```python
from build123d import *

# Parameters (mm, degrees)
SKETCH3_W             = 152.4
SKETCH3_H             = 152.4
BOSS_EXTRUDE3_DEPTH   = 3.175
SKETCH13_R            = 7.5
CUT_EXTRUDE5_DEPTH    = 4.175
SKETCH15_R            = 1
CUT_EXTRUDE6_DEPTH    = 4.175
SKETCH17_W            = 12
SKETCH17_H            = 10.5
CUT_EXTRUDE7_DEPTH    = 4.175
FILLET1_R             = 3
SKETCH19_R            = 1.05
CUT_EXTRUDE8_DEPTH    = 4.175
SKETCH20_R            = 2.9718
BOLT_HOLES_DEPTH      = 1
BOLT_HOLES_DEPTH_BACK = 4.175
CUT_EXTRUDE12_DEPTH   = 3.175
FILLET2_R             = 6.35
MIRROR5_COPY_1_DEPTH  = 3.175
FILLET3_R             = 6.35
FILLET4_R             = 6.35


with BuildPart() as part:
    # Sketch3 → Boss-Extrude3 (new body)
    with BuildSketch(Plane.XY):
        Rectangle(SKETCH3_W, SKETCH3_H)
    extrude(amount=BOSS_EXTRUDE3_DEPTH)

    # Sketch13 → Cut-Extrude5 (cut, through all)
    with BuildSketch(Plane(origin=(0.106889783, -2.03090588, 3.175), x_dir=(1, 0, 0), z_dir=(0, 0, 1))):
        Circle(SKETCH13_R)
    extrude(amount=-CUT_EXTRUDE5_DEPTH, mode=Mode.SUBTRACT)

    # Sketch15 → Cut-Extrude6 (cut, through all)
    with BuildSketch(Plane(origin=(0.106889783, -2.03090588, 3.175), x_dir=(1, 0, 0), z_dir=(0, 0, 1))):
        with Locations((-28.5, -28.5)):
            Circle(SKETCH15_R)
        with Locations((-28.5, 28.5)):
            Circle(SKETCH15_R)
        with Locations((28.5, -28.5)):
            Circle(SKETCH15_R)
        with Locations((28.5, 28.5)):
            Circle(SKETCH15_R)
    extrude(amount=-CUT_EXTRUDE6_DEPTH, mode=Mode.SUBTRACT)

    # Sketch17 → Cut-Extrude7 (cut, through all)
    with BuildSketch(Plane(origin=(0.106889783, -2.03090588, 3.175), x_dir=(1, 0, 0), z_dir=(0, 0, 1))):
        with Locations((6, 0.25)):
            Rectangle(SKETCH17_W, SKETCH17_H)
    extrude(amount=-CUT_EXTRUDE7_DEPTH, mode=Mode.SUBTRACT)

    # Fillet1
    fillet1_edges = [part.edges().sort_by_distance(p)[0] for p in [
        (12.106889783, -7.03090588, 1.5875),
        (12.106889783, 3.46909412, 1.5875),
    ]]
    fillet(fillet1_edges, radius=FILLET1_R)

    # Sketch19 → Cut-Extrude8 (cut, through all)
    with BuildSketch(Plane(origin=(0.106889783, -2.03090588, 3.175), x_dir=(1, 0, 0), z_dir=(0, 0, 1))):
        with Locations((6.72, 6.72)):
            Circle(SKETCH19_R)
        with Locations((-6.72, 6.72)):
            Circle(SKETCH19_R)
        with Locations((-6.72, -6.72)):
            Circle(SKETCH19_R)
        with Locations((6.72, -6.72)):
            Circle(SKETCH19_R)
        with Locations((0, 10)):
            Circle(SKETCH19_R)
        with Locations((-10, 0)):
            Circle(SKETCH19_R)
        with Locations((0, -10)):
            Circle(SKETCH19_R)
    extrude(amount=-CUT_EXTRUDE8_DEPTH, mode=Mode.SUBTRACT)

    # Sketch20 → Bolt Holes (cut, two sides)
    with BuildSketch(Plane.XY.offset(3.175)) as bolt_holes_sk:
        with Locations((-69.83, 69.83)):
            Circle(SKETCH20_R)
        with Locations((69.83, 69.83)):
            Circle(SKETCH20_R)
        with Locations((69.83, -69.83)):
            Circle(SKETCH20_R)
        with Locations((-69.83, -69.83)):
            Circle(SKETCH20_R)
    extrude(amount=BOLT_HOLES_DEPTH, mode=Mode.SUBTRACT)
    extrude(bolt_holes_sk.sketch, amount=-BOLT_HOLES_DEPTH_BACK, mode=Mode.SUBTRACT)

    # Sketch25 → Cut-Extrude12 (cut)
    with BuildSketch(Plane.XY.offset(3.175)):
        with BuildLine():
            Line((-76.2, 50.8), (-76.2, -50.8))
            ThreePointArc((-76.2, -50.8), (-46.628854397, 0), (-76.2, 50.8))
        make_face()
    cut_extrude12 = extrude(amount=-CUT_EXTRUDE12_DEPTH, mode=Mode.SUBTRACT)

    # Fillet2
    fillet2_edges = [part.edges().sort_by_distance(p)[0] for p in [
        (-76.2, -50.8, 1.5875),
        (-76.2, 50.8, 1.5875),
        (-76.2, -76.2, 1.5875),
        (-76.2, 76.2, 1.5875),
    ]]
    fillet(fillet2_edges, radius=FILLET2_R)

    # Mirror4: Cut-Extrude12 across plane
    add(cut_extrude12.mirror(Plane(origin=(0, 0, 0), x_dir=(0, 0, 1), z_dir=(0.707106781, -0.707106781, 0))), mode=Mode.SUBTRACT)

    # Mirror5: Cut-Extrude12 across plane
    add(cut_extrude12.mirror(Plane(origin=(0, 0, 0), x_dir=(0, 0, 1), z_dir=(-0.707106781, -0.707106781, 0))), mode=Mode.SUBTRACT)

    # Mirror5 copy 1 sketch → Mirror5 copy 1 (cut)
    with BuildSketch(Plane(origin=(0, 0, 3.175), x_dir=(-1, 0, 0), z_dir=(0, 0, 1))):
        with BuildLine():
            Line((-76.2, 50.8), (-76.2, -50.8))
            ThreePointArc((-76.2, -50.8), (-46.628854397, 0), (-76.2, 50.8))
        make_face()
    extrude(amount=-MIRROR5_COPY_1_DEPTH, mode=Mode.SUBTRACT)

    # Fillet3
    fillet3_edges = [part.edges().sort_by_distance(p)[0] for p in [
        (-50.8, -76.2, 1.5875),
        (50.8, -76.2, 1.5875),
        (76.2, 50.8, 1.5875),
        (76.2, -50.8, 1.5875),
        (76.2, -76.2, 1.5875),
        (76.2, 76.2, 1.5875),
    ]]
    fillet(fillet3_edges, radius=FILLET3_R)

    # Fillet4
    fillet4_edges = [part.edges().sort_by_distance(p)[0] for p in [
        (50.8, 76.2, 1.5875),
        (-50.8, 76.2, 1.5875),
    ]]
    fillet(fillet4_edges, radius=FILLET4_R)


solid = part.part
```
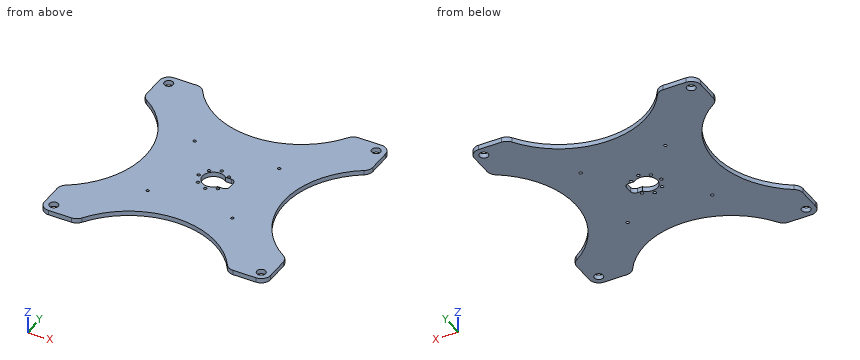
Work out the finished part from the listing and answer in its coordinate system (mm). Give positions to 0.01 mm unless a question says otherwise; leave off trailing zeros. Loops run counter-clockwise (first coordinate to the right, second up) from the corner with the lowest first, then second, coordinate; pieces in that order, holes last. Notation, with made-up numbers: (-16.5, -5.5) - (-4.5, -5.5) arc R22 ccw to (-4.5, 11.5) - close; hole circle Ø5 at (-27.5, 37). An arc over 180 degrees is marked (long way). Use CSV: the item, a comma, the result in double quotes. Start each with the question number.
(1) Find the intervals of material crossed by L1, parallel to Y at x = 6.5, z = 0.3; L2, parallel to X at y = 26, z = 2.25; L3, parallel to X at y = -69, z = 1.45, in increasing order.
(2) Each of these flat-tipped pins is pushed along its axis until it touches: pin 1 (3.5 mm diameter, centred on x = -69.83, y = -69.83, fed in from -Z); pin 2 (1 mm diameter, centred on y = -1.5, z = 2, fed in from -X). Where does it stop, or does it pass through?
(3) Find section D-D, the plane z = 0.5. Count the separate pieces of the cut face and the enclosed holes in it, plus the area to 3 significant figures.
(4) Find section A-A, the plane y = -63. Determine the outline of the cut face in (x, z) (3 decimals), plus the area to 3 significant figures.
(5) Find section C-C, the plane y = -24.5. Determine the outline of the cut face in (x, z) (3 decimals), plus the area to 3 significant figures.
(6) Find section B-B, the plane x = -51. Determine the outline of the cut face in (y, z) (3 decimals), plus the area to 3 significant figures.
Results found:
1,L1,"-46.99 to -9.75, -7.75 to -7.03, 3.47 to 3.69, 5.69 to 46.99"
1,L2,"-52.73 to -29.28, -27.51 to 27.72, 29.49 to 52.73"
1,L3,"-76.2 to -72.68, -66.98 to -45.97, 45.97 to 66.98, 72.68 to 76.2"
2,pin 1,"through"
2,pin 2,"x = -46.66"
3,separate pieces,"1"
3,enclosed holes,"16"
3,area,"14,300 mm^2"
4,outline,"(-76.2, 0) - (-40.556, 0) - (-40.556, 3.175) - (-76.2, 3.175) - close; (40.556, 0) - (76.2, 0) - (76.2, 3.175) - (40.556, 3.175) - close"
4,area,"226 mm^2"
5,outline,"(-52.014, 0) - (52.014, 0) - (52.014, 3.175) - (-52.014, 3.175) - close"
5,area,"330 mm^2"
6,outline,"(-75.231, 0) - (-22.172, 0) - (-22.172, 3.175) - (-75.231, 3.175) - close; (22.172, 0) - (75.231, 0) - (75.231, 3.175) - (22.172, 3.175) - close"
6,area,"337 mm^2"
